Part model, mm, in its own coordinate system. A direction names the side the tool comes from. Give positions to 0.01 mm unless a question says otherwise; leave off trailing zeros. Write each loop counter-clockwise with the first axis right and the second up, starting at its lowest first coordinate (ties: lowest second). Pieces come first, ordered by that corner, then holes. Notation, with made-up numbers: (49.5, 0) - (55.5, 0) arc R36 cw to (55.5, 35) - close; hole circle Ø10 at (68.5, -17). An arc over 180 degrees is marked (long way). Answer as a JSON object with one key per item and string values. Group by question number.
```python
from build123d import *

# Parameters (mm, degrees)
SKETCH1_R           = 28.575
BOSS_EXTRUDE1_DEPTH = 38.1


with BuildPart() as part:
    # Sketch1 → Boss-Extrude1 (new body)
    with BuildSketch(Plane(origin=(0, 0, 0), x_dir=(0, 0, -1), z_dir=(1, 0, 0))):
        with Locations(Location((0, 0, 0), (0, 0, 180))):
            Circle(SKETCH1_R)
        with BuildLine():
            ThreePointArc((12.7, 0), (-7.777129933, -10.040231571), (-3.175, 12.296722124))
            Line((-3.175, 12.296722124), (-3.175, 15.875))
            Line((-3.175, 15.875), (3.175, 15.875))
            Line((3.175, 15.875), (3.175, 12.296722124))
            ThreePointArc((3.175, 12.296722124), (10.040231571, 7.777129933), (12.7, 0))
        make_face(mode=Mode.SUBTRACT)
    extrude(amount=BOSS_EXTRUDE1_DEPTH)

    # Sketch2 → Cut-Revolve1 (revolve, cut)
    with BuildSketch(Plane.XY, mode=Mode.PRIVATE) as cut_revolve1_sk:
        Polygon((0, 28.575), (3.175, 28.575), (6.930717855, 18.25625), (12.119282145, 18.25625), (15.875, 28.575), (19.05, 28.575), (22.805717855, 18.25625), (27.994282145, 18.25625), (31.75, 28.575), (34.925, 28.575), (34.925, 3.709633234), (38.1, 3.709633234), (38.1, 28.575), (38.1, 34.001656794), (0, 34.001656794), align=None)
    revolve(cut_revolve1_sk.sketch.rotate(Axis((-1.262943143, 0, 0), (-1, 0, 0)), 270), axis=Axis((-1.262943143, 0, 0), (-1, 0, 0)), mode=Mode.SUBTRACT)


solid = part.part
```
1) Saw through at B-B (y = 24.5). State how many separate pieces and enclosed holes the cut face has, and give its area (3 significant figures).
2) Saw through at D-D (x = 15). List the corners of the cut face in (y, z) (3 decimals), and give its area (3 significant figures).
3) Saw through at C-C (x = 31). List the corners of the cut face in (y, z) (3 decimals), and give its area (3 significant figures).
4) Which spindle directions (+Z, -Z, +X, -X, +Y, -Y) get a long thin tool onto all of the face, cutting with end or side? Do faces 5 (the flat face through (0, 6, 12)), 6 (the conical face through (22.623, -18.311, -4.066)), 7 (the flat face through (17, 14, -3.175)). Say none if no direction does.
5) Drop flat-ended pins along their axis: P1, Ø5, axis at x = 31, z = 8.5, coming from the -Y side; P2, Ø1, axis at x = 16, y = -14, coming from the +Z side; P3, Ø4, axis at x = 31, z = 0, coming from the -Y side (3 decimals). Give the stop position or say it passes through.
6) Two-plate mould, pull along Z, no slides. Class faces 1 (the flat face through (17, 15.875, 0)), 2 (the flat face through (17, 14, 3.175)), 3 (the flat face through (34.925, -12, 6)), 4 (the conical face through (28.23, 5.68, 18.03)): +Z half, -Z half, draft (parallel to the pull), parting line (faces both ways), or undercut.
7) Drill centre lines: line 1 along Y through (x, z) = (25, 0) (3 decimals); line 2 along X through (y, z) = (3, 20.5) (3 decimals); line 3 along X through (y, z) = (-23, 11) (3 decimals). Where is each one in solid material? Low to high. Write a range as from..to.
8) Saw through at A-A (z = 0). List the corners of the cut face in (x, y) (3 decimals), and give its area (3 significant figures).
Checks:
{
 "1": {"separate pieces": "3", "enclosed holes": "0", "area": "395 mm2"},
 "2": {"outline": "circle Ø52.342 at (0, 0); hole (12.297, -3.175) - (15.875, -3.175) - (15.875, 3.175) - (12.297, 3.175) arc R12.7 ccw (long way) to start", "area": "1,620 mm2"},
 "3": {"outline": "circle Ø53.029 at (0, 0); hole (12.297, -3.175) - (15.875, -3.175) - (15.875, 3.175) - (12.297, 3.175) arc R12.7 ccw (long way) to start", "area": "1,680 mm2"},
 "4": {"face 5": "+Z, -Z, -X, +Y, -Y", "face 6": "none", "face 7": "+X, -X"},
 "5": {"P1": "y = -27.91", "P2": "z = 25.18", "P3": "y = -28.575"},
 "6": {"face 1": "undercut", "face 2": "undercut", "face 3": "draft", "face 4": "parting line"},
 "7": {"line 1": "-18.256..-12.7, 15.875..18.256", "line 2": "0..6.035, 13.015..21.91, 28.89..34.925", "line 3": "0..4.296, 14.754..20.171, 30.629..34.925"},
 "8": {"outline": "(0, -28.575) - (3.175, -28.575) - (6.931, -18.256) - (12.119, -18.256) - (15.875, -28.575) - (19.05, -28.575) - (22.806, -18.256) - (27.994, -18.256) - (31.75, -28.575) - (34.925, -28.575) - (34.925, -12.7) - (0, -12.7) - close; (0, 15.875) - (34.925, 15.875) - (34.925, 28.575) - (31.75, 28.575) - (27.994, 18.256) - (22.806, 18.256) - (19.05, 28.575) - (15.875, 28.575) - (12.119, 18.256) - (6.931, 18.256) - (3.175, 28.575) - (0, 28.575) - close", "area": "629 mm2"}
}
